Autodesk Inventor part; units mm, degrees
ref_plane "YZ Plane" through (0, 0, 0) normal (1, 0, 0) x (0, 1, 0)
ref_plane "XZ Plane" through (0, 0, 0) normal (0, 1, 0) x (-1, 0, 0)
ref_plane "XY Plane" through (0, 0, 0) normal (0, 0, 1) x (1, 0, 0)
sketch "スケッチ1" plane through (0, 0, 0) normal (0, 0, 1) x (1, 0, 0)
  line L0 (0, 0) -> (70, 0)
  line L1 (70, 0) -> (70, 120)
  line L2 (70, 120) -> (0, 120)
  line L3 (0, 120) -> (0, 0)
  dimension "d0" = 70
  dimension "d1" = 120
extrude "押し出し1" add sketch "スケッチ1" along normal blind 5
sketch "スケッチ2" plane through (0, 0, 5) normal (0, 0, 1) x (1, 0, 0)
  line L0 (0, 120) -> (0, 0)
  line L1 (0, 0) -> (70, 0)
  point P0 (35, 40)
  dimension "d4" = 35
  dimension "d5" = 40
hole "穴1" at (35, 40, 5) direction (0, 0, -1) diameter 12 end through all
sketch "スケッチ3" plane through (0, 0, 5) normal (0, 0, 1) x (1, 0, 0)
  circle A0 centre (35, 40) radius 6
  point P0 (0, 0)
  point P1 (34.9431, 14)
  point P2 (57.5451, 52.9507)
  point P3 (12.5118, 53.0493)
  dimension "d13" = 26
  dimension "d16" = 360
hole "穴2" at (34.9431, 14, 5) at (35, 40, 5) at (57.5451, 52.9507, 5) at (12.5118, 53.0493, 5) direction (0, 0, -1) diameter 3.5 end through all
sketch "スケッチ4" plane through (0, 0, 5) normal (0, 0, 1) x (1, 0, 0)
  line L0 (0, 120) -> (0, 0)
  line L1 (0, 0) -> (70, 0)
  point P0 (35, 40)
  point P1 (35, 58)
  point P2 (19.4115, 31)
  point P3 (50.5885, 31)
  dimension "d27" = 35
  dimension "d28" = 40
  dimension "d29" = 18
  dimension "d32" = 360
hole "穴3" at (35, 40, 5) at (35, 58, 5) at (19.4115, 31, 5) at (50.5885, 31, 5) direction (0, 0, -1) diameter 3.5 end through all
sketch "スケッチ6" plane through (0, 0, 5) normal (0, 0, 1) x (1, 0, 0)
  line L0 (0, 120) -> (0, 0)
  line L1 (0, 0) -> (70, 0)
  point P0 (35, 40)
  point P1 (10, 110)
  point P2 (60, 110)
  point P3 (10, 90)
  point P4 (60, 90)
  dimension "d43" = 35
  dimension "d44" = 40
  dimension "d48" = 110
  dimension "d49" = 110
  dimension "d50" = 90
  dimension "d51" = 90
hole "穴4" at (35, 40, 5) at (10, 110, 5) at (60, 110, 5) at (10, 90, 5) at (60, 90, 5) direction (0, 0, -1) diameter 5.5 end through all
properties part number "エンコーダ取り付け板"
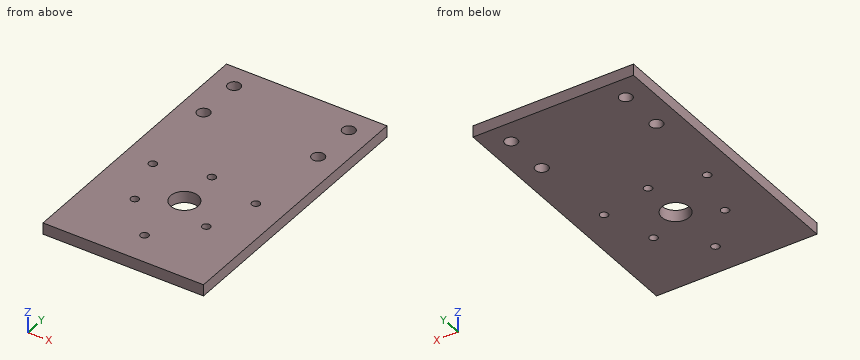
The model under review builds one solid part; all positions refer to its coordinate system, in mm. Round coordinates to 2 decimals unless told otherwise and drop trailing zeros. Write each loop counter-clockwise with the first axis right and the second up, starting at its lowest first coordinate (ties: lowest second). Pieces come first, ordered by that corner, then holes. Notation, with made-up numbers: M -29,63 L 17,63 A21 cw 17,77 Z; hole C 1,8.5 d1. An arc over 180 degrees is marked long. Use CSV: the item, a comma, the result in double quotes. Start each with the question number.
(1) We need section A-A, the plane y = 40. State the section outline as (x, z) points, then the cut area to 3 significant figures.
(2) We need section B-B, the plane y = 110. State the section outline as (x, z) points.
(3) We need section C-C, the plane z = 2.85. State how many separate pieces and enclosed holes the cut face has, then the cut area to 3 significant figures.
(4) For line 1 along Y through (x, z) = (60, 2.55); line 2 along Y through (x, z) = (35, 1.95); line 3 along X through (y, z) = (110, 2.8), list the stretches that pass through material, from the lowest coordinate up.
(5) We need section D-D, the plane y = 14. State the section outline as (x, z) points, then the cut area to 4 significant figures.
(6) Clearance check with flat-ended pins moving along their axes: P1, Ø3, axis at x = 19.41, y = 31, coming from the +Z side; P2, Ø6.5, axis at x = 60, y = 90, coming from the +Z side. State where each tip first meets the part, or that it passes through.
Findings:
1,outline,"M 0,0 L 29,0 L 29,5 L 0,5 Z; M 41,0 L 70,0 L 70,5 L 41,5 Z"
1,area,"290 mm^2"
2,outline,"M 0,0 L 7.25,0 L 7.25,5 L 0,5 Z; M 12.75,0 L 57.25,0 L 57.25,5 L 12.75,5 Z; M 62.75,0 L 70,0 L 70,5 L 62.75,5 Z"
3,separate pieces,"1"
3,enclosed holes,"11"
3,area,"8,130 mm^2"
4,line 1,"0 to 87.25, 92.75 to 107.25, 112.75 to 120"
4,line 2,"0 to 12.25, 15.75 to 34, 46 to 56.25, 59.75 to 120"
4,line 3,"0 to 7.25, 12.75 to 57.25, 62.75 to 70"
5,outline,"M 0,0 L 33.19,0 L 33.19,5 L 0,5 Z; M 36.69,0 L 70,0 L 70,5 L 36.69,5 Z"
5,area,"332.5 mm^2"
6,P1,"through"
6,P2,"z = 5"
